Source: CAD feature listing. Evaluate the final solid. Frame: model axes, mm. A direction names the side the tool comes from. Give positions to 0.01 mm unless a question says otherwise; leave off trailing zeros. Order: outer loops, then holes, each group sorted by start corner. A loop starts at its lowest first (then second) coordinate and runs counter-clockwise, first axis right, second up. Notation, with made-up numbers: M -23.5,-25 L -1.5,-25 A29 cw -1.5,-2 Z; hole C 61,41.25 d11. An arc over 180 degrees is marked long. Use CSV: the item, a comma, the result in double quotes. Start each with the question number.
1. Section query D-D, the plane x = 24. Return the cut outline in (y, z), plus the area to 3 significant figures.
2. Section query A-A, the plane z = 1.5. Return the cut outline in (x, y).
3. Mould query, pull axis Y, two halves, no side actions, for faces 1 (the flat face through (0, 0, 0)), 2 (the flat face through (15, 2.5, -1)), 3 (the flat face through (32, 0, 3.4)). Classes: released by +Y, released by -Y, zero draft, split by the parting line, or undercut.
4. Section query B-B, the plane y = 2. Return the cut outline in (x, z).
5. Reachability of faces 4 (the cylindrical face through (28.5, 0.07, 1.68)), 5 (the flat face through (0, -2, 6.8)) from +Z, -Z, +X, -X, +Y, -Y: full face, straight path, thin tool, end or side. Return the list, or none.
6. Section query C-C, the plane z = 4.5. Return the cut outline in (x, y).
7. Pin query (flat end, axial travel): P1, Ø1, axis at y = -0.5, z = 4.5, coming from the +X side; P2, Ø1, axis at x = 16.5, y = 1, coming from the +Z side. Return the tip coordinate at first contact, or that it passes through.
8. Line query: line 1 along Y through (x, z) = (30, 1.1); line 2 along X through (y, z) = (-1.3, 2); line 3 along X through (y, z) = (1.2, 0.5). Output: solid intervals per line, ascending. Write a range as [from, to].
from build123d import *

# Parameters (mm, degrees)
F0_R     = 2.5
F0_R_2   = 1.5
F1_DEPTH = 6.8
F2_R     = 1.5
F3_DEPTH = 1.2
F4_R     = 2.5
F4_R_2   = 1.5
F5_DEPTH = 3.4


with BuildPart() as f1:
    # F0 (on Top) → F1 (new body)
    with BuildSketch(Plane.XY):
        Circle(F0_R)
        Circle(F0_R_2, mode=Mode.SUBTRACT)
    extrude(amount=F1_DEPTH)

    # F2 (on face) → F3 (join)
    with BuildSketch(Plane(origin=(0, 0, 0), x_dir=(1, 0, 0), z_dir=(0, 0, -1))):
        with BuildLine():
            ThreePointArc((30, -2.5), (31.767767, -1.767767), (32.5, 0))
            ThreePointArc((32.5, 0), (31.767767, 1.767767), (30, 2.5))
            ThreePointArc((30, 2.5), (27.5, 0), (30, -2.5))
        make_face()
        with BuildLine():
            ThreePointArc((2.5, 0), (1.767767, 1.767767), (0, 2.5))
            ThreePointArc((0, 2.5), (-2.5, 0), (0, -2.5))
            ThreePointArc((0, -2.5), (1.767767, -1.767767), (2.5, 0))
        make_face()
        Circle(F2_R, mode=Mode.SUBTRACT)
        Circle(F2_R)
        with BuildLine():
            Line((30, 2.5), (0, 2.5))
            ThreePointArc((0, 2.5), (1.767767, 1.767767), (2.5, 0))
            ThreePointArc((2.5, 0), (1.767767, -1.767767), (0, -2.5))
            Line((0, -2.5), (30, -2.5))
            ThreePointArc((30, -2.5), (27.5, 0), (30, 2.5))
        make_face()
    extrude(amount=F3_DEPTH)

    # F4 (on face) → F5 (join)
    with BuildSketch(Plane.XY):
        with Locations((30, 0)):
            Circle(F4_R)
        with Locations((30, 0)):
            Circle(F4_R_2, mode=Mode.SUBTRACT)
    extrude(amount=F5_DEPTH)


solid = f1.part
Result set:
1,outline,"M -2.5,-1.2 L 2.5,-1.2 L 2.5,0 L -2.5,0 Z"
1,area,"6.00 mm2"
2,outline,"C 0,0 d5; C 30,0 d5; hole C 0,0 d3; hole C 30,0 d3"
3,face 1,"undercut"
3,face 2,"released by +Y"
3,face 3,"zero draft"
4,outline,"M -1.5,-1.2 L 31.5,-1.2 L 31.5,3.4 L 28.5,3.4 L 28.5,0 L 1.5,0 L 1.5,6.8 L -1.5,6.8 Z"
5,face 4,"+Z"
5,face 5,"+Z, +X, -X, +Y, -Y"
6,outline,"C 0,0 d5; hole C 0,0 d3"
7,P1,"x = 2.5"
7,P2,"z = 0"
8,line 1,"[-2.5, -1.5], [1.5, 2.5]"
8,line 2,"[-2.14, -0.75], [0.75, 2.14], [27.86, 29.25], [30.75, 32.14]"
8,line 3,"[-2.19, -0.9], [0.9, 2.19], [27.81, 29.1], [30.9, 32.19]"
